Geometry: see drawing. Coordinates: mm, zero at the bounding-box minimum. A direction names the side the tool comes from. Give positions to 0.01 mm unless a question says otherwise; leave off trailing zeros. Order: outer loops, then holes, each group sorted by start corner. A loop starts at its lowest first (then second) coordinate and runs counter-clockwise, first axis right, second up. Notation, with made-up numbers: (-27, 4) - (-5, 4) arc R30 ccw to (-5, 33) - close; hole circle Ø7 at (0.5, 60.25). An arc over 180 degrees is marked (long way). Put each result on its own line as item: value. Start each with the question number.
1. Section C-C on y = 1.05. Count the separate pieces of the cut face and the enclosed holes in it, plus the area to 3 significant figures.
2. Section B-B on z = 6. Return the cut outline in (x, y).
3. Set-up query: the marked faces 1 and 2. Return all of +Z, -Z, +X, -X, +Y, -Y with unobstructed straight access to the full face (end or side cutting, diameter ignored); none if empty.
4. Mould query, pull axis X, two halves, no side actions, for the marked faces 3, 4 and 5. Classes: pulls with the +X half, pulls with the -X half, needs draft (parallel to the pull), parting line crosses it, or undercut.
5. Section A-A on x = 10.5. Return the cut outline in (y, z).
6. Ray query, line 1 along X through (y, z) = (2.2, 3.75); line 2 along X through (y, z) = (0.9, 11) (1 decimal); line 3 along Z through (x, y) = (5.25, 1.95). Return the intervals inside material, ascending. Write a range as from..to.
7. Section D-D on z = 12.25. Return the cut outline in (x, y).
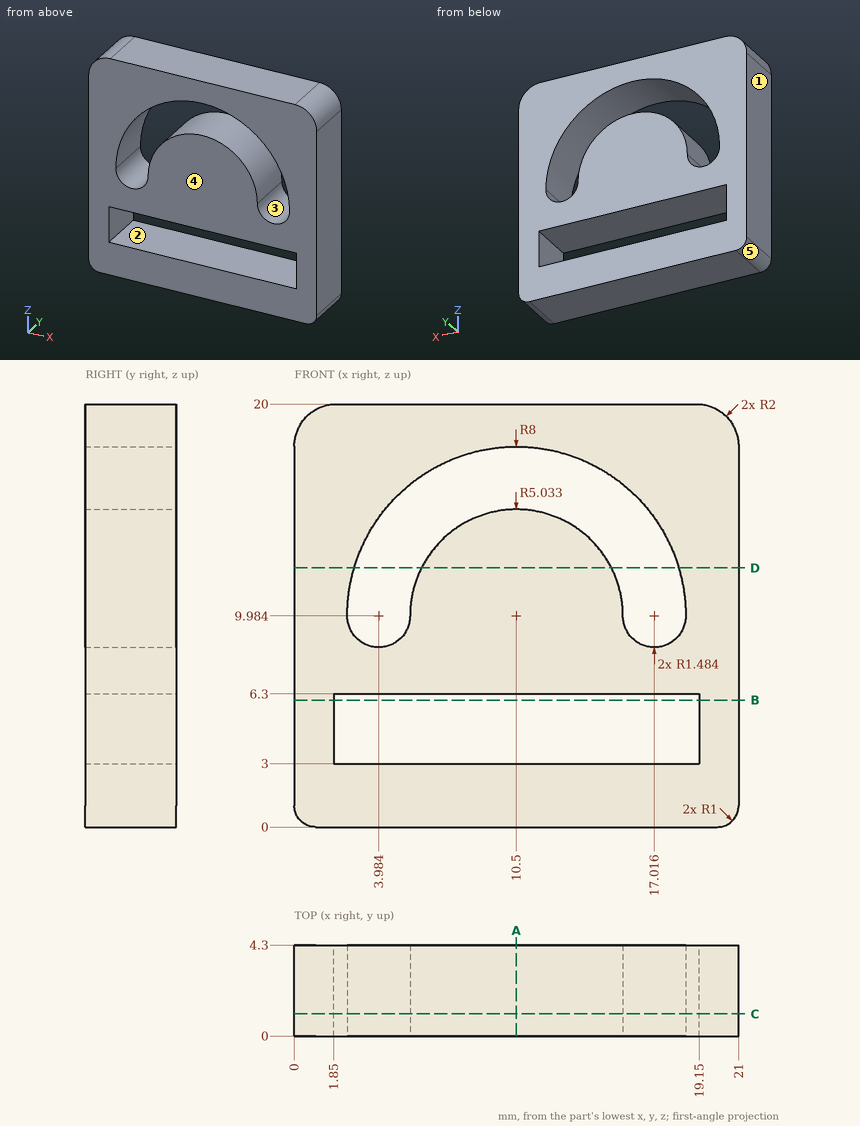
Resolved:
1. separate pieces: 1
1. enclosed holes: 2
1. area: 293 mm^2
2. outline: (0, 0) - (1.85, 0) - (1.85, 4.3) - (0, 4.3) - close; (19.15, 0) - (21, 0) - (21, 4.3) - (19.15, 4.3) - close
3. face 1: +Z, -Z, -X, +Y, -Y
3. face 2: +Y, -Y
4. face 3: undercut
4. face 4: needs draft
4. face 5: pulls with the -X half
5. outline: (0, 0) - (4.3, 0) - (4.3, 3) - (0, 3) - close; (0, 6.3) - (4.3, 6.3) - (4.3, 15.02) - (0, 15.02) - close; (0, 17.98) - (4.3, 17.98) - (4.3, 20) - (0, 20) - close
6. line 1: 0..1.85, 19.15..21
6. line 2: 0..2.6, 5.6..15.4, 18.4..21
6. line 3: 0..3, 6.3..9.21, 16.02..20
7. outline: (0, 0) - (2.83, 0) - (2.83, 4.3) - (0, 4.3) - close; (6.01, 0) - (14.99, 0) - (14.99, 4.3) - (6.01, 4.3) - close; (18.17, 0) - (21, 0) - (21, 4.3) - (18.17, 4.3) - close
